```python
from build123d import *

# Parameters (mm, degrees)
CROQUIS1_W                       = 57.15
CROQUIS1_H                       = 31.75
BRIDA_BASE1_DEPTH                = 2.667
BRIDA_DE_ARISTA1_STRIP_W         = 11.684
BRIDA_DE_ARISTA1_STRIP_H         = 2.667
BRIDA_DE_ARISTA1_STRIP_CUT_DEPTH = 57.15
BRIDA_DE_ARISTA1_DEPTH           = 57.15
CROQUIS9_R                       = 3.937
CORTAR_EXTRUIR1_DEPTH            = 5.588
CROQUIS10_R                      = 2.667
CORTAR_EXTRUIR2_DEPTH            = 5.588


# Sheet-metal steps are written as plain solids
with BuildPart() as part:
    # Croquis1 → Brida base1 (new body)
    with BuildSketch(Plane.XY):
        Rectangle(CROQUIS1_W, CROQUIS1_H)
    extrude(amount=-BRIDA_BASE1_DEPTH)

    # Brida de arista1 strip (across the edge) → Brida de arista1 strip cut (cut)
    with BuildSketch(Plane(origin=(-28.575, 15.875, -2.667), x_dir=(0, -1, 0), z_dir=(1, 0, 0))):
        with Locations((-2.667, -1.3335)):
            Rectangle(BRIDA_DE_ARISTA1_STRIP_W, BRIDA_DE_ARISTA1_STRIP_H)
    extrude(amount=BRIDA_DE_ARISTA1_STRIP_CUT_DEPTH, mode=Mode.SUBTRACT)

    # Brida de arista1 section (across the edge) → Brida de arista1 (add)
    with BuildSketch(Plane(origin=(-28.575, 15.875, -2.667), x_dir=(0, -1, 0), z_dir=(1, 0, 0))):
        with BuildLine():
            Line((0, 0.508), (0, 30.353))
            Line((0, 30.353), (2.667, 30.353))
            Line((2.667, 30.353), (2.667, 0.508))
            ThreePointArc((2.667, 0.508), (2.815789755, 0.148789755), (3.175, 0))
            Line((3.175, 0), (3.175, -2.667))
            ThreePointArc((3.175, -2.667), (0.92993597, -1.73706403), (0, 0.508))
        make_face()
    extrude(amount=BRIDA_DE_ARISTA1_DEPTH)

    # Croquis9 → Cortar-Extruir1 (cut)
    with BuildSketch(Plane.XY):
        with Locations((-21.463, -3.175)):
            Circle(CROQUIS9_R)
        with Locations((21.463, -3.175)):
            Circle(CROQUIS9_R)
    extrude(amount=-CORTAR_EXTRUIR1_DEPTH, mode=Mode.SUBTRACT)

    # Croquis10 → Cortar-Extruir2 (cut)
    with BuildSketch(Plane(origin=(0, 15.875, 0), x_dir=(1, 0, 0), z_dir=(0, 1, 0))):
        with Locations(Location((0, 23.368, 0), (0, 0, 270))):
            Circle(CROQUIS10_R)
        Polygon((-28.575, 33.02), (-8.001, 33.02), (-28.575, 12.446), align=None)
        Polygon((28.575, 33.02), (8.001, 33.02), (28.575, 12.446), align=None)
    extrude(amount=-CORTAR_EXTRUIR2_DEPTH, mode=Mode.SUBTRACT)


solid = part.part
```
Part model, mm, in its own coordinate system. A direction names the side the tool comes from. Round coordinates to 2 decimals unless told otherwise and drop trailing zeros. Loops run counter-clockwise (first coordinate to the right, second up) from the corner with the lowest first, then second, coordinate; pieces in that order, holes last.
Item 1: Cut at D-D, the plane y = 6. Give the cut face in (x, z) (3 decimals), then the cut area to 3 significant figures.
Item 2: Cut at C-C, the plane z = -14. Give the cut face in (x, y) (3 decimals).
Item 3: Cut at B-B, the plane x = 21. Give the cut face in (y, z) (3 decimals), then the cut area to 3 significant figures.
Item 4: Cut at A-A, the plane x = 0. Give the cut face in (y, z) (3 decimals).
Item 5: Drop flat-ended pins along their axis: P1, Ø6.5, axis at x = 21.463, y = -3.175, coming from the -Z side; P2, Ø4, axis at x = 18.5, y = 5, coming from the -Z side; P3, Ø5, axis at x = 8.5, z = -21.5, coming from the -Y side. Give the stop position or say it passes through.
Item 6: Drill centre lines: line 1 (Z direction, x = 18, y = 9); line 2 (Y direction, x = -2, z = -13.5) (3 decimals); line 3 (Y direction, x = 18, z = -2.5) (3 decimals). Where is each one in solid material? Low to high.
Item 7: 3-axis set-ups, long thin cutter, end or side, ignore diameter. For faces 4 (the face through (0, -1, -2.667)), 5 (the face through (0, 15, -33.02)): which of +Z, -Z, +X, -X, +Y, -Y reach the whole face in a straight line?
Item 8: Mould opens along X. For faces 1 (the face through (0, -1, 0)), 2 (the face through (25.1, -4.68, -1.31)), 3 (the face through (18.14, 14.56, -22.88)) say: +X half, -X half, draft (parallel to the pull), parting line (faces both ways), or undercut.
A:
1. outline: (-28.575, -2.667) - (28.575, -2.667) - (28.575, 0) - (-28.575, 0) - close
1. area: 152 mm2
2. outline: (-27.021, 13.208) - (27.021, 13.208) - (27.021, 15.875) - (-27.021, 15.875) - close
3. outline: (-15.875, -2.667) - (-7.085, -2.667) - (-7.085, 0) - (-15.875, 0) - close; (0.735, -2.667) - (12.7, -2.667) arc R0.508 cw to (13.208, -3.175) - (13.208, -20.021) - (15.875, -20.021) - (15.875, -3.175) arc R3.175 ccw to (12.7, 0) - (0.735, 0) - close
3. area: 108 mm2
4. outline: (-15.875, -2.667) - (12.7, -2.667) arc R0.508 cw to (13.208, -3.175) - (13.208, -20.701) - (15.875, -20.701) - (15.875, -3.175) arc R3.175 ccw to (12.7, 0) - (-15.875, 0) - close; (13.208, -33.02) - (15.875, -33.02) - (15.875, -26.035) - (13.208, -26.035) - close
5. P1: passes through
5. P2: stops at z = -2.67
5. P3: stops at y = 13.21
6. line 1: z = -2.67 to 0
6. line 2: y = 13.208 to 15.875
6. line 3: y = -15.875 to -5.048, -1.302 to 15.802
7. face 4: -Z, +X, -X, -Y
7. face 5: -Z, +X, -X, +Y, -Y
8. face 1: draft
8. face 2: undercut
8. face 3: +X half
